Source: CAD feature listing. Evaluate the final solid. Frame: model axes, mm. A direction names the side the tool comes from. Coordinates: 2 decimals unless noted, no trailing zeros. Write each loop counter-clockwise with the first axis right and the second up, starting at its lowest first coordinate (ties: lowest second). Pieces come first, ordered by that corner, then holes. Notation, with made-up numbers: M -12,-35.5 L 42,-35.5 A24 cw 42,-1.5 Z; hole C -4,-36 d8. An arc over 180 degrees is marked long. One line per item, written item: value. Start each with the question number.
Item 1: Cut plane C-C, the plane z = -26. Output: boundary loops of the cut face in (x, y), then the cut area to 3 significant figures.
Item 2: Pin query (flat end, axial travel): P1, Ø10, axis at x = -11.5, z = 11, coming from the -Y side; P2, Ø13, axis at x = 5, z = 1, coming from the -Y side; P3, Ø1.5, axis at x = -16, y = 6, coming from the -Z side; P4, Ø2, axis at y = 7, z = 20.5, coming from the -X side. Return the tip coordinate at first contact, or that it passes through.
Item 3: Ray query, L1, parallel to X at y = 6.2, z = 0; L2, parallel to Z at x = 0, y = 3.85; L3, parallel to X at y = 0.75, z = 0.5. Return the intervals inside material, ascending. Write a range as from..to.
Item 4: Set-up query: faces 1 (the cylindrical face through (10.846, 4.043, -18.733)), 2 (the cylindrical face through (-10.158, 2.766, 7.789)). Return all of +Z, -Z, +X, -X, +Y, -Y with unobstructed straight access to the full face (end or side cutting, diameter ignored); none if empty.
Item 5: Cut plane B-B, the plane y = 6.5. State how many separate pieces and enclosed holes the cut face has, then the cut area to 3 significant figures.
Item 6: Cut plane A-A, the plane x = 17. Output: boundary loops of the cut face in (y, z).
Item 7: Mould query, pull axis Z, two halves, no side actions, for faces 3 (the cylindrical face through (-29.97, 4.16, -1.32)), 4 (the flat face through (-7, 8.2, 0)), 5 (the flat face through (-3, 5.2, -6)). Classes: released by +Z, released by -Z, zero draft, split by the parting line, or undercut.
Item 8: Cut plane D-D, the plane x = 0. Output: boundary loops of the cut face in (y, z), then the cut area to 3 significant figures.
```python
from build123d import *

# Parameters (mm, degrees)
SKETCH001_R  = 5.5
POCKET_DEPTH = 8.201
CHAMFER_SIZE = 0.4


with BuildPart() as part:
    # Sketch → Revolution (revolve)
    with BuildSketch(Plane.XY):
        Polygon((30, 0), (30, 8.2), (6.3, 8.2), (6.3, 5.2), (12.8, 5.2), (12.8, 0), align=None)
    revolve(axis=Axis((0, 0, 0), (0, 1, 0)))

    # Sketch001 (on Face6 of Revolution) → Pocket (cut, through all)
    with BuildSketch(Plane.XZ):
        with Locations((0.124373, 21.635731)):
            Circle(SKETCH001_R)
        with Locations((15.386717, 15.210827)):
            Circle(SKETCH001_R)
        with Locations((21.635731, -0.124373)):
            Circle(SKETCH001_R)
        with Locations((15.210827, -15.386717)):
            Circle(SKETCH001_R)
        with Locations((-0.124373, -21.635731)):
            Circle(SKETCH001_R)
        with Locations((-15.386717, -15.210827)):
            Circle(SKETCH001_R)
        with Locations((-21.635731, 0.124373)):
            Circle(SKETCH001_R)
        with Locations((-15.210827, 15.386717)):
            Circle(SKETCH001_R)
    extrude(amount=-POCKET_DEPTH, mode=Mode.SUBTRACT)

    # Chamfer
    chamfer_edges = [part.edges().sort_by_distance(p)[0] for p in [
        (-12.8, 0, 0),
    ]]
    chamfer(chamfer_edges, length=CHAMFER_SIZE)


solid = part.part
```
From the geometry:
1. outline: M -14.97,0 L -3.47,0 L -3.47,8.2 L -14.97,8.2 Z; M 3.22,0 L 14.97,0 L 14.97,8.2 L 3.22,8.2 Z
1. area: 191 mm²
2. P1: stops at y = 0
2. P2: stops at y = 5.2
2. P3: stops at z = -25.83
2. P4: stops at x = -22.8
3. L1: x = -30..-27.13, -16.14..-6.3, 6.3..16.14, 27.13..30
3. L2: z = -30..-27.13, -16.14..-12.8, 12.8..16.14, 27.13..30
3. L3: x = -30..-27.12, -16.15..-12.79, 12.79..16.17, 27.1..30
4. face 1: +Y, -Y
4. face 2: -Y
5. separate pieces: 1
5. enclosed holes: 9
5. area: 1,940 mm²
6. outline: M 0,-24.72 L 8.2,-24.72 L 8.2,-20.59 L 0,-20.59 Z; M 0,-10.19 L 8.2,-10.19 L 8.2,-3.08 L 0,-3.08 Z; M 0,2.84 L 8.2,2.84 L 8.2,9.95 L 0,9.95 Z; M 0,20.47 L 8.2,20.47 L 8.2,24.72 L 0,24.72 Z
7. face 3: split by the parting line
7. face 4: zero draft
7. face 5: undercut
8. outline: M 0,-30 L 8.2,-30 L 8.2,-27.13 L 0,-27.13 Z; M 0,-16.14 L 8.2,-16.14 L 8.2,-6.3 L 5.2,-6.3 L 5.2,-12.8 L 0.4,-12.8 L 0,-13.2 Z; M 0,13.2 L 0.4,12.8 L 5.2,12.8 L 5.2,6.3 L 8.2,6.3 L 8.2,16.14 L 0,16.14 Z; M 0,27.13 L 8.2,27.13 L 8.2,30 L 0,30 Z
8. area: 141 mm²
